Input: dimensioned drawing with shaded views. Units: mm. Origin: part minimum x, y, z. A direction names the side the tool comes from. Round coordinates to 2 decimals unless told otherwise and drop trailing zeros. Order: outer loops, then holes, each group sorted by start corner. A loop starts at its lowest first (then second) coordinate and runs counter-clockwise, first axis right, second up. Notation, with made-up numbers: M 36.5,-17.5 L 44.5,-17.5 A19 ccw 44.5,17.5 Z; hole C 29.25,-21.75 d3. An arc over 180 degrees is marked long. Put each result on its own line as item: value. Start each with the question number.
1) First-contact query: P1, Ø4, axis at x = 13.5, y = 132.5, coming from the -Z side; P2, Ø20, axis at x = 27.5, z = 198, coming from the +Y side; P3, Ø4, axis at y = 102.5, z = 151.5, coming from the -X side; P4, Ø1.5, axis at x = 59.5, y = 88, coming from the -Z side. Flat tips, straight axial feed; report the tip coordinate or a pass-through.
2) Access query for the marked faces 1, 2, 3, 4 and 5. Directions: +Z, -Z, +X, -X, +Y, -Y. A direction counts if a zero-diameter tool reaches every point of the face in a straight line with its end or side. Return the directions, or none.
3) Section A-A, the plane y = 33. Return loops of the section in (x, z).
4) Section C-C, the plane z = 191.5. Return loops of the section in (x, y).
5) Draft query along Z for the marked faces 6, 7 and 8. Return one class per face: pulls with the +Z half, pulls with the -Z half, needs draft (parallel to the pull), parting line crosses it, or undercut.
6) Material intervals for probe 1 along Z at (x, y) = (6.5, 117); probe 2 along Z at (x, y) = (8, 39); probe 3 along Z at (x, y) = (12.5, 64), sorted ascending. Write a range as [from, to].
7) Section B-B, the plane x = 88. Return loops of the section in (y, z), then the cut area to 3 significant figures.
8) Section D-D, the plane y = 80.5. Return loops of the section in (x, z), then the cut area to 3 significant figures.
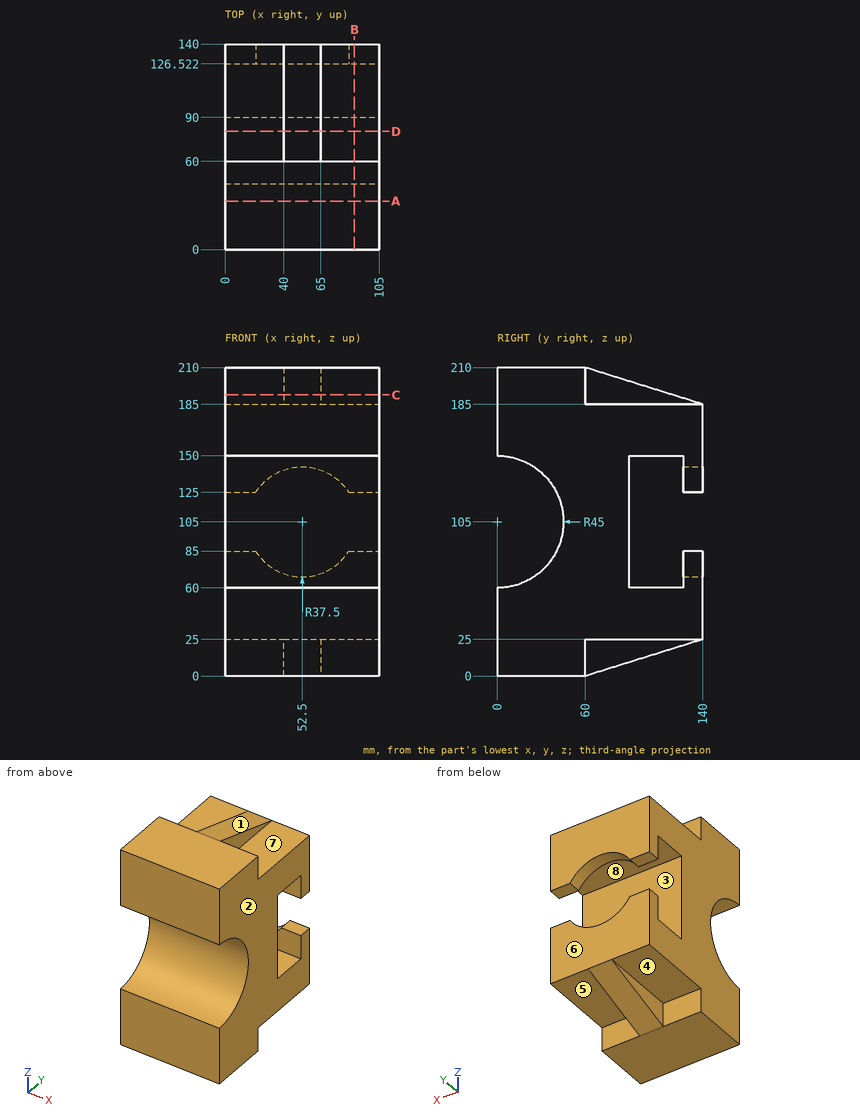
Result sheet:
1. P1: stops at z = 25
1. P2: stops at y = 60
1. P3: stops at x = 0
1. P4: stops at z = 8.52
2. face 1: +Z, +X, -X, +Y
2. face 2: +Z, -Z, +X, +Y, -Y
2. face 3: +X, -X
2. face 4: -Z, -X, +Y
2. face 5: -Z, +X, +Y
3. outline: M 0,0 L 105,0 L 105,74.41 L 0,74.41 Z; M 0,135.59 L 105,135.59 L 105,210 L 0,210 Z
4. outline: M 0,0 L 105,0 L 105,60 L 65,60 L 65,119.2 L 40,119.2 L 40,60 L 0,60 Z
5. face 6: needs draft
5. face 7: pulls with the +Z half
5. face 8: undercut
6. probe 1: z = [25, 60], [150, 185]
6. probe 2: z = [0, 82.55], [127.45, 210]
6. probe 3: z = [25, 185]
7. outline: M 0,0 L 60,0 L 60,25 L 140,25 L 140,85 L 126.52,85 L 126.52,60 L 90,60 L 90,150 L 126.52,150 L 126.52,125 L 140,125 L 140,185 L 60,185 L 60,210 L 0,210 L 0,150 A45 cw 0,60 Z
7. area: 18,400 mm2
8. outline: M 0,25 L 40,25 L 40,6.41 L 65,6.41 L 65,25 L 105,25 L 105,185 L 65,185 L 65,203.59 L 40,203.59 L 40,185 L 0,185 Z
8. area: 17,700 mm2
